Autodesk Inventor part; units mm, degrees
ref_plane "YZ Plane" through (0, 0, 0) normal (1, 0, 0) x (0, 1, 0)
ref_plane "XZ Plane" through (0, 0, 0) normal (0, 1, 0) x (-1, 0, 0)
ref_plane "XY Plane" through (0, 0, 0) normal (0, 0, 1) x (1, 0, 0)
sketch "Sketch1" plane through (0, 0, 0) normal (0, 1, 0) x (-1, 0, 0)
  line L0 (-279.4, -127.4986) -> (-279.4, -151.8986)
  line L1 (-277.4, -125.4986) -> (-174.3, -125.4986)
  line L2 (-174.3, -153.8986) -> (-277.4, -153.8986)
  circle A0 centre (-275.8, -47.0543) radius 1.25
  circle A1 centre (-261, -47.0543) radius 1.25
  circle A2 centre (-246.2, -47.0543) radius 1.25
  circle A3 centre (-261, -232.44) radius 1.25
  circle A4 centre (-18.4, -47.0543) radius 1.25
  circle A5 centre (-48.23, -117.9957) radius 1.778
  circle A6 centre (-48.23, -162.1917) radius 1.778
  circle A7 centre (-105.38, -162.1917) radius 1.778
  circle A8 centre (-105.38, -117.9957) radius 1.778
  line L3 (0, 0) -> (-279.4, 0)
  line L4 (-279.4, 0) -> (-279.4, -279.4)
  line L5 (-279.4, -279.4) -> (0, -279.4)
  line L6 (0, -279.4) -> (0, 0)
  line L7 (-279.4, 0) -> (-228.6, 0)
  line L8 (-228.6, 0) -> (-228.6, -41.275)
  line L9 (-228.6, -41.275) -> (-279.4, -41.275)
  line L10 (-279.4, -41.275) -> (-279.4, 0)
  line L11 (-279.4, -279.4) -> (-228.6, -279.4)
  line L12 (-228.6, -279.4) -> (-228.6, -238.125)
  line L13 (-228.6, -238.125) -> (-279.4, -238.125)
  line L14 (-279.4, -238.125) -> (-279.4, -279.4)
  line L15 (0, -279.4) -> (-50.8, -279.4)
  line L16 (-50.8, -279.4) -> (-50.8, -238.125)
  line L17 (-50.8, -238.125) -> (0, -238.125)
  line L18 (0, -238.125) -> (0, -279.4)
  line L19 (0, 0) -> (-50.8, 0)
  line L20 (-50.8, 0) -> (-50.8, -41.275)
  line L21 (-50.8, -41.275) -> (0, -41.275)
  line L22 (0, -41.275) -> (0, 0)
  arc A9 (-174.3, -153.6986) -> (-174.3, -125.6986) centre (-182.3, -139.6986) ccw
  line L23 (-162.35, -123.8236) -> (-289.35, -123.8236)
  line L24 (-289.35, -123.8236) -> (-289.35, -155.5736)
  line L25 (-289.35, -155.5736) -> (-162.35, -155.5736)
  line L26 (-162.35, -155.5736) -> (-162.35, -123.8236)
  line L27 (-162.35, -123.8236) -> (-289.35, -155.5736) construction
  line L28 (-289.35, -123.8236) -> (-162.35, -155.5736) construction
  line L29 (-280.05, -238.79) -> (-241.95, -238.79)
  line L30 (-241.95, -238.79) -> (-241.95, -226.09)
  line L31 (-241.95, -226.09) -> (-280.05, -226.09)
  line L32 (-280.05, -226.09) -> (-280.05, -238.79)
  line L33 (-280.05, -238.79) -> (-241.95, -226.09) construction
  line L34 (-241.95, -238.79) -> (-280.05, -226.09) construction
  circle A10 centre (-261, -232.44) radius 1.5875
  circle A11 centre (-246.2, -232.44) radius 1.5875
  circle A12 centre (-275.8, -232.44) radius 1.5875
  line L35 (-261, -47.0543) -> (-261, -232.44)
  line L36 (-261, -232.44) -> (-18.4, -232.44)
  circle A13 centre (-261, -47.0454) radius 1.5875
  line L37 (-280.05, -53.3954) -> (-241.95, -53.3954)
  line L38 (-241.95, -53.3954) -> (-241.95, -40.6954)
  line L39 (-241.95, -40.6954) -> (-280.05, -40.6954)
  circle A14 centre (-246.2, -47.0454) radius 1.5875
  line L40 (-280.05, -40.6954) -> (-280.05, -53.3954)
  circle A15 centre (-275.8, -47.0454) radius 1.5875
  circle A16 centre (-18.4046, -232.44) radius 1.5875
  line L41 (-37.4546, -238.79) -> (0.6454, -238.79)
  line L42 (0.6454, -238.79) -> (0.6454, -226.09)
  line L43 (0.6454, -226.09) -> (-37.4546, -226.09)
  circle A17 centre (-3.6046, -232.44) radius 1.5875
  line L44 (-37.4546, -226.09) -> (-37.4546, -238.79)
  circle A18 centre (-33.2046, -232.44) radius 1.5875
  circle A19 centre (-18.4046, -47.0454) radius 1.5875
  line L45 (-37.4546, -53.3954) -> (0.6454, -53.3954)
  line L46 (0.6454, -53.3954) -> (0.6454, -40.6954)
  line L47 (0.6454, -40.6954) -> (-37.4546, -40.6954)
  circle A20 centre (-3.6046, -47.0454) radius 1.5875
  line L48 (-37.4546, -40.6954) -> (-37.4546, -53.3954)
  circle A21 centre (-33.2046, -47.0454) radius 1.5875
  point P0 (-225.85, -139.6986)
  dimension "d4" = 279.4
  dimension "d5" = 279.4
  dimension "d6" = 50.8
  dimension "d7" = 41.275
  dimension "d8" = 50.8
  dimension "d9" = 41.275
  dimension "d10" = 50.8
  dimension "d11" = 41.275
  dimension "d12" = 41.275
  dimension "d13" = 127
  dimension "d14" = 31.75
  dimension "d15" = 38.1
  dimension "d16" = 12.7
  dimension "d17" = 3.175
  dimension "d18" = 185.3946
  dimension "d19" = 242.5954
extrude "Extrusion1" add sketch "Sketch1" along normal blind 12.7 contours L4 L23 L35 L25 L0 | L4 L37 L35 L23 | L25 L35 L31 L4 | L4 L9 L38 L37 | L35 L37 L38 L9 L8 L3 L20 L21 L48 L45 L6 L43 L44 L36 L30 L31 L25 L26 L23 | L23 L26 L25 L35 | L31 L35 A10 L36 A11 L30 L13 L4 | L31 L30 L36 A11 A10 L35 | L30 L36 L44 L17 L16 L5 L12 L13 | L44 L43 L6 L17 | L21 L6 L45 L48
sketch "Sketch3" plane through (0, 0, 0) normal (0, 1, 0) x (-1, 0, 0)
  line L0 (-279.4, -127.4986) -> (-279.4, -151.8986)
  line L1 (-277.4, -125.4986) -> (-174.3, -125.4986)
  line L2 (-174.3, -153.8986) -> (-277.4, -153.8986)
  circle A0 centre (-246.2, -47.0543) radius 1.25
  circle A1 centre (-261, -232.44) radius 1.25
  circle A2 centre (-18.4, -47.0543) radius 1.25
  circle A3 centre (-48.23, -117.9957) radius 1.778
  circle A4 centre (-48.23, -162.1917) radius 1.778
  circle A5 centre (-105.38, -162.1917) radius 1.778
  circle A6 centre (-105.38, -117.9957) radius 1.778
  line L3 (0, 0) -> (-279.4, 0)
  line L4 (-279.4, 0) -> (-279.4, -279.4)
  line L5 (-279.4, -279.4) -> (0, -279.4)
  line L6 (0, -279.4) -> (0, 0)
  line L7 (-279.4, 0) -> (-228.6, 0)
  line L8 (-279.4, -41.275) -> (-279.4, 0)
  line L9 (-279.4, -279.4) -> (-228.6, -279.4)
  line L10 (-228.6, -279.4) -> (-228.6, -238.125)
  line L11 (-228.6, -238.125) -> (-279.4, -238.125)
  line L12 (-279.4, -238.125) -> (-279.4, -279.4)
  line L13 (0, -279.4) -> (-50.8, -279.4)
  line L14 (-50.8, -279.4) -> (-50.8, -238.125)
  line L15 (-50.8, -238.125) -> (0, -238.125)
  line L16 (0, -238.125) -> (0, -279.4)
  line L17 (0, 0) -> (-50.8, 0)
  line L18 (-50.8, 0) -> (-50.8, -41.275)
  line L19 (-50.8, -41.275) -> (0, -41.275)
  line L20 (0, -41.275) -> (0, 0)
  arc A7 (-174.3, -153.6986) -> (-174.3, -125.6986) centre (-182.3, -139.6986) ccw
  line L21 (-162.35, -123.8236) -> (-289.35, -123.8236)
  line L22 (-289.35, -123.8236) -> (-289.35, -155.5736)
  line L23 (-289.35, -155.5736) -> (-162.35, -155.5736)
  line L24 (-162.35, -155.5736) -> (-162.35, -123.8236)
  line L25 (-162.35, -123.8236) -> (-289.35, -155.5736) construction
  line L26 (-289.35, -123.8236) -> (-162.35, -155.5736) construction
  line L27 (-280.05, -238.79) -> (-241.95, -238.79)
  line L28 (-241.95, -238.79) -> (-241.95, -226.09)
  line L29 (-241.95, -226.09) -> (-280.05, -226.09)
  line L30 (-280.05, -226.09) -> (-280.05, -238.79)
  line L31 (-280.05, -238.79) -> (-241.95, -226.09) construction
  line L32 (-241.95, -238.79) -> (-280.05, -226.09) construction
  circle A8 centre (-261, -232.44) radius 1.5875
  circle A9 centre (-246.2, -232.44) radius 1.5875
  circle A10 centre (-275.8, -232.44) radius 1.5875
  line L33 (-261, -47.0543) -> (-261, -232.44)
  line L34 (-261, -232.44) -> (-18.4, -232.44)
  circle A11 centre (-261, -47.0454) radius 1.5875
  line L35 (-280.05, -53.3954) -> (-241.95, -53.3954)
  line L36 (-241.95, -53.3954) -> (-241.95, -40.6954)
  line L37 (-241.95, -40.6954) -> (-280.05, -40.6954)
  circle A12 centre (-246.2, -47.0454) radius 1.5875
  line L38 (-280.05, -40.6954) -> (-280.05, -53.3954)
  circle A13 centre (-275.8, -47.0454) radius 1.5875
  circle A14 centre (-18.4046, -232.44) radius 1.5875
  line L39 (-37.4546, -238.79) -> (0.6454, -238.79)
  line L40 (0.6454, -238.79) -> (0.6454, -226.09)
  line L41 (0.6454, -226.09) -> (-37.4546, -226.09)
  circle A15 centre (-3.6046, -232.44) radius 1.5875
  line L42 (-37.4546, -226.09) -> (-37.4546, -238.79)
  circle A16 centre (-33.2046, -232.44) radius 1.5875
  circle A17 centre (-18.4046, -47.0454) radius 1.5875
  line L43 (-37.4546, -53.3954) -> (0.6454, -53.3954)
  line L44 (0.6454, -53.3954) -> (0.6454, -40.6954)
  line L45 (0.6454, -40.6954) -> (-37.4546, -40.6954)
  circle A18 centre (-3.6046, -47.0454) radius 1.5875
  line L46 (-37.4546, -40.6954) -> (-37.4546, -53.3954)
  circle A19 centre (-33.2046, -47.0454) radius 1.5875
  point P0 (-225.85, -139.6986)
  dimension "d26" = 279.4
  dimension "d27" = 279.4
  dimension "d30" = 50.8
  dimension "d31" = 41.275
  dimension "d32" = 50.8
  dimension "d33" = 41.275
  dimension "d34" = 41.275
  dimension "d35" = 127
  dimension "d36" = 31.75
  dimension "d37" = 38.1
  dimension "d38" = 12.7
  dimension "d39" = 3.175
  dimension "d40" = 185.3946
  dimension "d41" = 242.5954
extrude "Extrusion2" cut sketch "Sketch3" along normal blind 1.5875 contours L4 L21 L33 L23 L0 | L0 L4 L23 L22 L21 | L35 L38 L37 L4 | L4 L37 L36 L35 | L21 L24 L23 L33 | L29 L33 A8 L34 A9 L28 L11 L4 | L4 L27 L30 L29 | L11 L28 L27 L4 | L29 L28 L34 A9 A8 L33 | L42 L41 L6 L15 | L15 L6 L39 L42 | L41 L40 L39 L6 | L45 L44 L43 L6 | L6 L19 L46 L45 | L19 L6 L43 L46
properties part number "BottomPlateV1" material "Wood (Birch)"
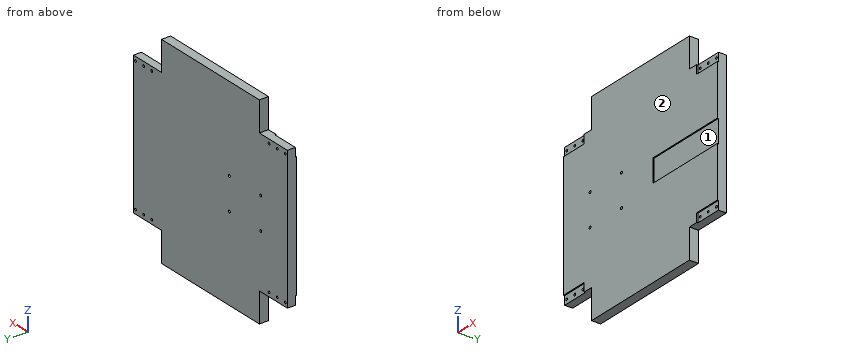
Check sheet for the modelled part. Datum: model origin and axes. Units: mm. Face numbers are marked on the shaded views. Round coordinates to 2 decimals unless told otherwise and drop trailing zeros. Write each loop counter-clockwise with the first axis right and the second up, starting at its lowest first coordinate (ties: lowest second). Pieces come first, ordered by that corner, then holes. Notation, with made-up numbers: (-19, 6) - (17, 6) arc R13 ccw to (17, 18) - close; hole circle Ø9 at (-17.5, 46.5). An arc over 180 degrees is marked (long way). Return JSON: item names as keys, results as strings.
Q1. Cross-section at A-A (y = 5.75). Give the number of separate pieces and of enclosed holes in the cut face, then the cut area to 3 significant figures.
Returned:
{"separate pieces": "1", "enclosed holes": "16", "area": "69,500 mm²"}
Q2. Cross-section at C-C (z = -246.5). Record the boundary of the cut face in (x, y).
Returned:
{"outline": "(50.8, 0) - (228.6, 0) - (228.6, 12.7) - (50.8, 12.7) - close"}
Q3. Scan lines: L1, parallel to Z at x = 48.23, y = 3.25 (3 decimals); L2, parallel to Z at x = 246.2, y = 6 (1 decimal); L3, parallel to X at y = 3.75, z = -163.5. Record each from-to range of solid material in increasing order. Write a range as from..to.
Returned:
{"L1": "z = -238.125..-163.97, -160.414..-119.774, -116.218..-41.275", "L2": "z = -238.1..-234, -230.9..-48.6, -45.5..-41.3", "L3": "x = 0..47.03, 49.43..104.18, 106.58..279.4"}
Q4. Depth check by flat-ended pin: P1, Ø0.8, axis at x = 259, y = 0.5, coming from the +Z side; P2, Ø1.7, axis at x = 21, y = 1, coming from the +Z side (3 decimals); P3, Ø6.5, axis at y = 7.5, z = -27, coming from the -X side. Enter the tip coordinate at first touch or a pass-through.
Returned:
{"P1": "stops at z = -53.4", "P2": "stops at z = -41.275", "P3": "stops at x = 50.8"}
Q5. Cross-section at B-B (x = 42). Record the boundary of the cut face in (y, z) (3 decimals), then the cut area to 3 significant figures.
Returned:
{"outline": "(0, -238.125) - (12.7, -238.125) - (12.7, -41.275) - (0, -41.275) - close", "area": "2,500 mm²"}
Q6. Draft check along Z on the marked faces 1 and 2. Enter one of: released by +Z, released by -Z, zero draft, split by the parting line, or undercut.
Returned:
{"face 1": "undercut", "face 2": "zero draft"}
